Geometry: final body of the model. Coordinates: model frame, mm. Face numbers are marked on the shaded views. A direction names the side the tool comes from. Give positions to 0.01 mm unless a question says otherwise; leave off trailing zeros. Order: outer loops, then holes, each group sorted by start corner. A loop starts at its lowest first (then second) coordinate and runs counter-clockwise, first axis right, second up. Notation, with made-up numbers: M -3.5,76 L 54.5,76 A12 ccw 54.5,99 Z; hole C -14,-14.5 d11. An arc over 180 degrees is marked long. Use CSV: the item, a comma, the result in double quotes.
Autodesk Inventor part; units mm, degrees
ref_plane "YZ Plane" through (0, 0, 0) normal (1, 0, 0) x (0, 1, 0)
ref_plane "XZ Plane" through (0, 0, 0) normal (0, 1, 0) x (-1, 0, 0)
ref_plane "XY Plane" through (0, 0, 0) normal (0, 0, 1) x (1, 0, 0)
sketch "スケッチ1" plane through (0, 0, 0) normal (0, 0, 1) x (1, 0, 0)
  line L0 (-24, 43) -> (24, 43)
  line L1 (24, 43) -> (24, -43)
  line L2 (24, -43) -> (-24, -43)
  line L3 (-24, -43) -> (-24, 43)
  point P0 (0, 0)
  point P1 (0, 43)
  point P2 (24, 0)
  dimension "d0" = 48
  dimension "d1" = 86
extrude "押し出し1" add sketch "スケッチ1" along normal blind 1.6
sketch "スケッチ2" plane through (0, 0, 1.6) normal (0, 0, 1) x (1, 0, 0)
  line L0 (-23.75, 34.8) -> (23.75, 34.8)
  line L1 (23.75, 34.8) -> (23.75, -34.8)
  line L2 (23.75, -34.8) -> (-23.75, -34.8)
  line L3 (-23.75, -34.8) -> (-23.75, 34.8)
  point P0 (0, 0)
  point P1 (0, 34.8)
  point P2 (23.75, 0)
  dimension "d4" = 47.5
  dimension "d5" = 69.6
extrude "押し出し2" add sketch "スケッチ2" along normal blind 12
sketch "スケッチ3" plane through (0, 0, 1.6) normal (0, 0, 1) x (1, 0, 0)
  line L0 (-24, -43) -> (24, -43)
  line L1 (-24, 43) -> (-24, -43)
  line L2 (24, -43) -> (24, 43)
  line L3 (24, 43) -> (-24, 43)
  circle A0 centre (-20, -39) radius 1.5
  circle A1 centre (20, -39) radius 1.5
  circle A2 centre (-20, 39) radius 1.5
  circle A3 centre (20, 39) radius 1.5
  point P0 (0, 0)
  dimension "d8" = 4
  dimension "d9" = 4
  dimension "d10" = 4
  dimension "d11" = 4
  dimension "d12" = 3
extrude "押し出し3" cut sketch "スケッチ3" against normal blind 1.6 contours A0 | A1 | A2 | A3
sketch "スケッチ4" plane through (0, 0, 13.6) normal (0, 0, 1) x (1, 0, 0)
  line L0 (-19.4086, 28.472) -> (45.9399, 28.472) construction
  line L1 (45.9399, 28.472) -> (45.9399, -30.0693) construction
  line L2 (45.9399, -30.0693) -> (-19.4086, -30.0693) construction
  line L3 (-19.4086, -30.0693) -> (-19.4086, 28.472) construction
  point P0 (0, 0)
properties part number "Big7seg"
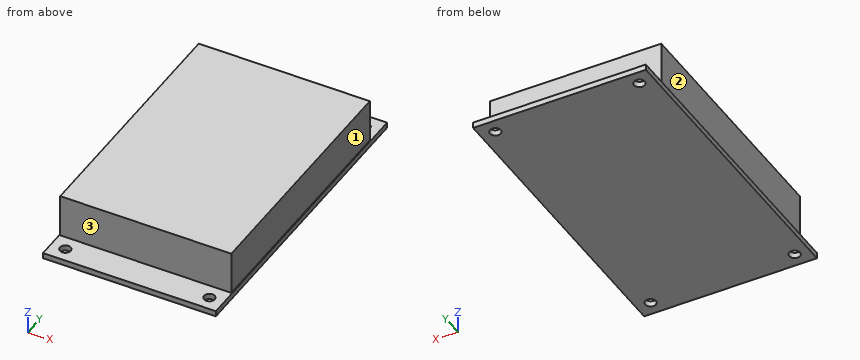
1. Section C-C, the plane x = -8.5. Return the cut outline in (y, z), plus the area to 3 significant figures.
Answer:
outline,"M -43,0 L 43,0 L 43,1.6 L 34.8,1.6 L 34.8,13.6 L -34.8,13.6 L -34.8,1.6 L -43,1.6 Z"
area,"973 mm2"
2. Reachability of the marked faces 1, 2 and 3 from +Z, -Z, +X, -X, +Y, -Y: full face, straight path, thin tool, end or side. Return the list, or none.
Answer:
face 1,"+Z, +X, +Y, -Y"
face 2,"+Z, -X, +Y, -Y"
face 3,"+Z, +X, -X, -Y"
3. Pin query (flat end, axial travel): pin 1 Ø3 at (x, z) = (-1, 7.5) entering from +Y; pin 2 Ø6 at (y, z) = (18, 8.5) entering from -X; pin 3 Ø4 at (y, z) = (-0.5, 5.5) entering from +X. Return the tip coordinate at first contact, or that it passes through.
Answer:
pin 1,"y = 34.8"
pin 2,"x = -23.75"
pin 3,"x = 23.75"
4. Section A-A, the plane x = 20. Return the cut outline in (y, z), plus the area to 3 significant figures.
Answer:
outline,"M -43,0 L -40.5,0 L -40.5,1.6 L -43,1.6 Z; M -37.5,0 L 37.5,0 L 37.5,1.6 L 34.8,1.6 L 34.8,13.6 L -34.8,13.6 L -34.8,1.6 L -37.5,1.6 Z; M 40.5,0 L 43,0 L 43,1.6 L 40.5,1.6 Z"
area,"963 mm2"
5. Line query: line 1 (Y direction, x = 20, z = 0.8); line 2 (X direction, y = 25.5, z = 11); line 3 (Y direction, x = -20, z = 3.25). Output: solid intervals per line, ascending.
Answer:
line 1,"-43 to -40.5, -37.5 to 37.5, 40.5 to 43"
line 2,"-23.75 to 23.75"
line 3,"-34.8 to 34.8"
6. Section B-B, the plane y = -39. Return the cut outline in (x, z), plus the area to 3 significant figures.
Answer:
outline,"M -24,0 L -21.5,0 L -21.5,1.6 L -24,1.6 Z; M -18.5,0 L 18.5,0 L 18.5,1.6 L -18.5,1.6 Z; M 21.5,0 L 24,0 L 24,1.6 L 21.5,1.6 Z"
area,"67.2 mm2"
7. Section D-D, the plane z = 12.25. Return the cut outline in (x, y), plus the area to 3 significant figures.
Answer:
outline,"M -23.75,-34.8 L 23.75,-34.8 L 23.75,34.8 L -23.75,34.8 Z"
area,"3,310 mm2"
